from build123d import *

# Parameters (mm, degrees)
SKETCH2_W           = 54
SKETCH2_H           = 162
SKETCH2_R           = 10
SKETCH2_R_2         = 10.5
BOSS_EXTRUDE1_DEPTH = 12
SKETCH3_W           = 18
SKETCH3_H           = 12
BOSS_EXTRUDE2_DEPTH = 12
CUT_EXTRUDE1_REACH  = 99.581
SKETCH4_R           = 2.25
LPATTERN1_COUNT     = 2
LPATTERN1_PITCH     = 90
CUT_EXTRUDE2_DEPTH  = 6
CUT_EXTRUDE3_REACH  = 99.581
SKETCH6_R           = 5
SKETCH8_R           = 5
CUT_EXTRUDE4_DEPTH  = 6
CUT_EXTRUDE5_REACH  = 99.026
SKETCH9_R           = 3
SKETCH10_R          = 3
CUT_EXTRUDE6_DEPTH  = 19
CUT_EXTRUDE7_REACH  = 99.581
SKETCH11_R          = 3
CUT_EXTRUDE8_DEPTH  = 6
CUT_EXTRUDE9_REACH  = 99.581
SKETCH13_R          = 2.5
CUT_EXTRUDE10_DEPTH = 6


with BuildPart() as part:
    # Sketch2 → Boss-Extrude1 (new body)
    with BuildSketch(Plane(origin=(0, 0, 0), x_dir=(0, 0, -1), z_dir=(1, 0, 0))):
        Rectangle(SKETCH2_W, SKETCH2_H)
        Circle(SKETCH2_R, mode=Mode.SUBTRACT)
        with Locations((0, 45)):
            Circle(SKETCH2_R_2, mode=Mode.SUBTRACT)
        with Locations((0, -45)):
            Circle(SKETCH2_R_2, mode=Mode.SUBTRACT)
    extrude(amount=BOSS_EXTRUDE1_DEPTH)

    # Sketch3 → Boss-Extrude2 (add)
    with BuildSketch(Plane(origin=(12, 0, 0), x_dir=(0, 0, -1), z_dir=(1, 0, 0))):
        with Locations((0, -87)):
            Rectangle(SKETCH3_W, SKETCH3_H)
    boss_extrude2 = extrude(amount=-BOSS_EXTRUDE2_DEPTH)

    # Mirror1: Boss-Extrude2 across plane
    add(boss_extrude2.mirror(Plane.ZX))

    # Sketch4 → Cut-Extrude1 (cut, up to next)
    with BuildSketch(Plane(origin=(12, 0, 0), x_dir=(0, 0, -1), z_dir=(1, 0, 0)), mode=Mode.PRIVATE) as cut_extrude1_sk1:
        with Locations((-16, -45)):
            Circle(SKETCH4_R)
    cut_extrude1_tool1 = extrude(cut_extrude1_sk1.sketch, amount=-CUT_EXTRUDE1_REACH, mode=Mode.PRIVATE) & part.part
    # Sketch4 → Cut-Extrude1 (cut, up to next)
    with BuildSketch(Plane(origin=(12, 0, 0), x_dir=(0, 0, -1), z_dir=(1, 0, 0)), mode=Mode.PRIVATE) as cut_extrude1_sk2:
        with Locations((16, -45)):
            Circle(SKETCH4_R)
    cut_extrude1_tool2 = extrude(cut_extrude1_sk2.sketch, amount=-CUT_EXTRUDE1_REACH, mode=Mode.PRIVATE) & part.part
    cut_extrude1_1 = cut_extrude1_tool1.solids().sort_by_distance((12, -45, 16))[0]
    add(cut_extrude1_1, mode=Mode.SUBTRACT)
    cut_extrude1_2 = cut_extrude1_tool2.solids().sort_by_distance((12, -45, -16))[0]
    add(cut_extrude1_2, mode=Mode.SUBTRACT)
    cut_extrude1 = cut_extrude1_1 + cut_extrude1_2  # Cut-Extrude1 as one shape, for the pattern or mirror that repeats it

    # LPattern1: Cut-Extrude1 ×2
    with Locations(*[(0, i * LPATTERN1_PITCH, 0) for i in range(1, LPATTERN1_COUNT)]):
        add(cut_extrude1, mode=Mode.SUBTRACT)

    # Sketch5 → Cut-Extrude2 (cut)
    with BuildSketch(Plane.ZY):
        with BuildLine():
            Line((16.992645468, 29.5), (-16.992645468, 29.5))
            ThreePointArc((-16.992645468, 29.5), (-23, 45), (-16.992645468, 60.5))
            Line((-16.992645468, 60.5), (16.992645468, 60.5))
            ThreePointArc((16.992645468, 60.5), (23, 45), (16.992645468, 29.5))
        make_face()
        with BuildLine():
            Line((16.992645468, -60.5), (-16.992645468, -60.5))
            ThreePointArc((-16.992645468, -60.5), (-23, -45), (-16.992645468, -29.5))
            Line((-16.992645468, -29.5), (16.992645468, -29.5))
            ThreePointArc((16.992645468, -29.5), (23, -45), (16.992645468, -60.5))
        make_face()
    extrude(amount=-CUT_EXTRUDE2_DEPTH, mode=Mode.SUBTRACT)

    # Sketch6 → Cut-Extrude3 (cut, up to next)
    with BuildSketch(Plane.ZY, mode=Mode.PRIVATE) as cut_extrude3_sk1:
        with Locations((-18, -69)):
            Circle(SKETCH6_R)
    cut_extrude3_tool1 = extrude(cut_extrude3_sk1.sketch, amount=-CUT_EXTRUDE3_REACH, mode=Mode.PRIVATE) & part.part
    # Sketch6 → Cut-Extrude3 (cut, up to next)
    with BuildSketch(Plane.ZY, mode=Mode.PRIVATE) as cut_extrude3_sk2:
        with Locations((18, -69)):
            Circle(SKETCH6_R)
    cut_extrude3_tool2 = extrude(cut_extrude3_sk2.sketch, amount=-CUT_EXTRUDE3_REACH, mode=Mode.PRIVATE) & part.part
    cut_extrude3_1 = cut_extrude3_tool1.solids().sort_by_distance((0, -69, -18))[0]
    add(cut_extrude3_1, mode=Mode.SUBTRACT)
    cut_extrude3_2 = cut_extrude3_tool2.solids().sort_by_distance((0, -69, 18))[0]
    add(cut_extrude3_2, mode=Mode.SUBTRACT)
    cut_extrude3 = cut_extrude3_1 + cut_extrude3_2  # Cut-Extrude3 as one shape, for the pattern or mirror that repeats it

    # Sketch8 → Cut-Extrude4 (cut)
    with BuildSketch(Plane.ZY):
        with Locations((0, -87)):
            Circle(SKETCH8_R)
    cut_extrude4 = extrude(amount=-CUT_EXTRUDE4_DEPTH, mode=Mode.SUBTRACT)

    # Sketch9 → Cut-Extrude5 (cut, up to next)
    with BuildSketch(Plane.ZY.offset(-6), mode=Mode.PRIVATE) as cut_extrude5_sk1:
        with Locations((0, -87)):
            Circle(SKETCH9_R)
    cut_extrude5_tool1 = extrude(cut_extrude5_sk1.sketch, amount=-CUT_EXTRUDE5_REACH, mode=Mode.PRIVATE) & part.part
    cut_extrude5 = cut_extrude5_tool1.solids().sort_by_distance((6, -87, 0))[0]
    add(cut_extrude5, mode=Mode.SUBTRACT)

    # Sketch10 → Cut-Extrude6 (cut)
    with BuildSketch(Plane.XZ.offset(81)):
        with Locations(Location((6, -18, 0), (0, 0, 270))):
            Circle(SKETCH10_R)
        with Locations(Location((6, 18, 0), (0, 0, 270))):
            Circle(SKETCH10_R)
    cut_extrude6 = extrude(amount=-CUT_EXTRUDE6_DEPTH, mode=Mode.SUBTRACT)

    # Sketch11 → Cut-Extrude7 (cut, up to next)
    with BuildSketch(Plane.ZY, mode=Mode.PRIVATE) as cut_extrude7_sk1:
        with Locations((-21, -22.5)):
            Circle(SKETCH11_R)
    cut_extrude7_tool1 = extrude(cut_extrude7_sk1.sketch, amount=-CUT_EXTRUDE7_REACH, mode=Mode.PRIVATE) & part.part
    cut_extrude7 = cut_extrude7_tool1.solids().sort_by_distance((0, -22.5, -21))[0]
    add(cut_extrude7, mode=Mode.SUBTRACT)

    # Sketch12 → Cut-Extrude8 (cut)
    with BuildSketch(Plane.ZY):
        with BuildLine():
            Line((-21, -27.5), (-27, -27.5))
            Line((-27, -27.5), (-27, -17.5))
            Line((-27, -17.5), (-21, -17.5))
            ThreePointArc((-21, -17.5), (-16, -22.5), (-21, -27.5))
        make_face()
    cut_extrude8 = extrude(amount=-CUT_EXTRUDE8_DEPTH, mode=Mode.SUBTRACT)

    # Mirror2: Cut-Extrude3, Cut-Extrude4, Cut-Extrude5, Cut-Extrude6, Cut-Extrude7, Cut-Extrude8 across plane
    add(cut_extrude3.mirror(Plane.ZX), mode=Mode.SUBTRACT)
    add(cut_extrude4.mirror(Plane.ZX), mode=Mode.SUBTRACT)
    add(cut_extrude5.mirror(Plane.ZX), mode=Mode.SUBTRACT)
    add(cut_extrude6.mirror(Plane.ZX), mode=Mode.SUBTRACT)
    add(cut_extrude7.mirror(Plane.ZX), mode=Mode.SUBTRACT)
    add(cut_extrude8.mirror(Plane.ZX), mode=Mode.SUBTRACT)

    # Sketch13 → Cut-Extrude9 (cut, up to next)
    with BuildSketch(Plane.ZY, mode=Mode.PRIVATE) as cut_extrude9_sk1:
        with Locations((0, 15)):
            Circle(SKETCH13_R)
    cut_extrude9_tool1 = extrude(cut_extrude9_sk1.sketch, amount=-CUT_EXTRUDE9_REACH, mode=Mode.PRIVATE) & part.part
    # Sketch13 → Cut-Extrude9 (cut, up to next)
    with BuildSketch(Plane.ZY, mode=Mode.PRIVATE) as cut_extrude9_sk2:
        with Locations((0, -15)):
            Circle(SKETCH13_R)
    cut_extrude9_tool2 = extrude(cut_extrude9_sk2.sketch, amount=-CUT_EXTRUDE9_REACH, mode=Mode.PRIVATE) & part.part
    add(cut_extrude9_tool1.solids().sort_by_distance((0, 15, 0))[0], mode=Mode.SUBTRACT)
    add(cut_extrude9_tool2.solids().sort_by_distance((0, -15, 0))[0], mode=Mode.SUBTRACT)

    # Sketch14 → Cut-Extrude10 (cut)
    with BuildSketch(Plane.ZY):
        with BuildLine():
            Line((-16, 12.816005618), (-16, -12.816005618))
            ThreePointArc((-16, -12.816005618), (20.5, 0), (-16, 12.816005618))
        make_face()
    extrude(amount=-CUT_EXTRUDE10_DEPTH, mode=Mode.SUBTRACT)


solid = part.part
Source: CAD feature listing. Evaluate the final solid. Frame: model axes, mm. A direction names the side the tool comes from. Give positions to 0.01 mm unless a question says otherwise; leave off trailing zeros. Order: outer loops, then holes, each group sorted by start corner. A loop starts at its lowest first (then second) coordinate and runs counter-clockwise, first axis right, second up. Notation, with made-up numbers: (26, -26) -> (40, -26) arc R4 cw to (40, -20) -> close; hole circle Ø5 at (29.5, -4.5). An arc over 180 degrees is marked (long way). Write item = value, one per line.
Q1. Cut plane B-B, the plane y = -22.5. Output: boundary loops of the cut face in (x, z), and give its area (3 significant figures).
Data:
outline = (0, -16) -> (6, -16) -> (6, -18) -> (12, -18) -> (12, 27) -> (0, 27) -> close; (6, -27) -> (12, -27) -> (12, -24) -> (6, -24) -> close
area = 546 mm^2
Q2. Set-up query: faces 1 (the face through (6, -4, 10)), 2 (the face through (3, -81, -20)), 3 (the face through (3, -81, 16)), 4 (the face through (3, -17.5, -24)), 5 (the face through (6, -77, 21)). Return all of +Z, -Z, +X, -X, +Y, -Y with unobstructed straight access to the full face (end or side cutting, diameter ignored); none if empty.
Data:
face_1 = -X
face_2 = -Z, +X, -X, -Y
face_3 = +Z, +X, -X, -Y
face_4 = -Z, -X
face_5 = -Y
Q3. Cut plane D-D, the plane y = 52. Output: boundary loops of the cut face in (x, z), and give its area (3 significant figures).
Data:
outline = (0, -27) -> (12, -27) -> (12, -7.83) -> (6, -7.83) -> (6, -21.91) -> (0, -21.91) -> close; (0, 21.91) -> (6, 21.91) -> (6, 7.83) -> (12, 7.83) -> (12, 27) -> (0, 27) -> close
area = 291 mm^2
Q4. Pull-direction query (Y, two-part tool) for faces 6 (the face through (3, -29.5, 0)), 7 (the face through (6, -87, 9)), 8 (the face through (6, 93, 0)); classes: released by +Y, released by -Y, zero draft, split by the parting line, or undercut.
Data:
face_6 = undercut
face_7 = zero draft
face_8 = released by +Y
Q5. Pin query (flat end, axial travel): pin 1 (5 mm diameter, centred on y = -89, z = -1, fed in from -X); pin 2 (5 mm diameter, centred on x = 4.5, z = -18.5, fed in from -Y); pin 3 (3 mm diameter, centred on x = 8, z = 13, fed in from +Y). Return the tip coordinate at first contact, or that it passes through.
Data:
pin_1 = 6
pin_2 = -81
pin_3 = 81
Q6. Cut plane A-A, the plane y = -87. Output: boundary loops of the cut face in (x, z), and give its area (3 significant figures).
Data:
outline = (0, -9) -> (12, -9) -> (12, -3) -> (6, -3) -> (6, -5) -> (0, -5) -> close; (0, 5) -> (6, 5) -> (6, 3) -> (12, 3) -> (12, 9) -> (0, 9) -> close
area = 120 mm^2
Q7. Material intervals for line 1 (Y direction, x = 7.25, z = -21); line 2 (Z direction, x = 3.25, y = 69); line 3 (Y direction, x = 5.75, z = -24), sorted ascending. Write a range as from..to.
Data:
line_1 = -81..-73, -65..-25.5, -19.5..19.5, 25.5..65, 73..81
line_2 = -27..-23, -13..13, 23..27
line_3 = -81..-27.5, -17.5..17.5, 27.5..81
Q8. Cut plane C-C, the plane z = 0.5. State how many separate pieces and enclosed holes the cut face has, and give its area (3 significant figures).
Data:
separate_pieces = 8
enclosed_holes = 0
area = 993 mm^2
